```python
from build123d import *

# Parameters (mm, degrees)
F0_W     = 165
F0_H     = 165
F1_DEPTH = 20
F2_R     = 21
F3_DEPTH = 80
F4_DEPTH = 20


with BuildPart() as f1:
    # F0 (on Top) → F1 (new body)
    with BuildSketch(Plane.XY):
        Rectangle(F0_W, F0_H)
    extrude(amount=F1_DEPTH)

    # F2 (on Top) → F3 (join)
    with BuildSketch(Plane.XY):
        with Locations((0, -39.440217)):
            Circle(F2_R)
    extrude(amount=F3_DEPTH)

    # F2 (on Top) → F4 (join)
    with BuildSketch(Plane.XY):
        with Locations((0, -39.440217)):
            Circle(F2_R)
    extrude(amount=-F4_DEPTH)


solid = f1.part
```
Source: CAD feature listing. Evaluate the final solid. Frame: model axes, mm. A direction names the side the tool comes from. Give positions to 0.01 mm unless a question says otherwise; leave off trailing zeros. Loops run counter-clockwise (first coordinate to the right, second up) from the corner with the lowest first, then second, coordinate; pieces in that order, holes last. Notation, with made-up numbers: (74.5, 2.5) -> (102.5, 2.5) arc R23 cw to (102.5, 27.5) -> close; hole circle Ø1 at (66.5, -35.75). An arc over 180 degrees is marked (long way). Put each result on its own line as item: value. Start each with the question number.
1) Cut plane D-D (x = 65.5). Return loops of the section in (y, z).
2) Draft query along Y for faces 3 (the face through (-82.5, -1, 10)), 4 (the face through (20.03, -33.13, 49.58)), 5 (the face through (-1, 82.5, 10)). Return one class per face: released by +Y, released by -Y, zero draft, split by the parting line, or undercut.
3) Cut plane A-A (x = 0). Return loops of the section in (y, z), then the cut area to 3 significant figures.
4) Material intervals for probe 1 along Z at (x, y) = (-27.5, -29.5); probe 2 along Y at (x, z) = (0, 32.5); probe 3 along X at (y, z) = (-38, 61), sorted ascending.
5) Cut plane B-B (y = -35.5). Return loops of the section in (x, z).
6) Contact query for flat-ended pins moving along their axis: P1, Ø12, axis at x = 7.5, z = 53, coming from the -Y side; P2, Ø3, axis at y = -29.5, z = 30, coming from the +X side; P3, Ø2, axis at y = -52, z = 56, coming from the -X side. Output: stop coordinate, or through.
7) Reachability of faces 1 (the face through (82.5, -1, 10)), 2 (the face through (20.03, -33.13, -9.86)) from +Z, -Z, +X, -X, +Y, -Y: full face, straight path, thin tool, end or side. Return the list, or none.
8) Cut plane C-C (z = 64). Return loops of the section in (x, y), then the cut area to 3 significant figures.
Results are:
1. outline: (-82.5, 0) -> (82.5, 0) -> (82.5, 20) -> (-82.5, 20) -> close
2. face 3: zero draft
2. face 4: split by the parting line
2. face 5: released by +Y
3. outline: (-82.5, 0) -> (-60.44, 0) -> (-60.44, -20) -> (-18.44, -20) -> (-18.44, 0) -> (82.5, 0) -> (82.5, 20) -> (-18.44, 20) -> (-18.44, 80) -> (-60.44, 80) -> (-60.44, 20) -> (-82.5, 20) -> close
3. area: 6,660 mm2
4. probe 1: z = 0 to 20
4. probe 2: y = -60.44 to -18.44
4. probe 3: x = -20.95 to 20.95
5. outline: (-82.5, 0) -> (-20.63, 0) -> (-20.63, -20) -> (20.63, -20) -> (20.63, 0) -> (82.5, 0) -> (82.5, 20) -> (20.63, 20) -> (20.63, 80) -> (-20.63, 80) -> (-20.63, 20) -> (-82.5, 20) -> close
6. P1: stops at y = -60.39
6. P2: stops at x = 19.23
6. P3: stops at x = -17.53
7. face 1: +Z, -Z, +X, +Y, -Y
7. face 2: -Z
8. outline: circle Ø42 at (0, -39.44)
8. area: 1,390 mm2
